Geometry: final body of the model. Coordinates: model frame, mm. A direction names the side the tool comes from. Round coordinates to 2 decimals unless told otherwise and drop trailing zeros. Write each loop counter-clockwise with the first axis right and the second up, starting at its lowest first coordinate (ties: lowest second). Pieces come first, ordered by that corner, then holes. Notation, with made-up numbers: M 42,-35 L 98,-35 A33 ccw 98,-2 Z; hole C 35.5,70 d9. An arc over 180 degrees is marked long. Answer as CSV lines item,"result". Start each with the question number.
Q1. Mould query, pull axis Y, two halves, no side actions, for faces 1 (the cylindrical face through (56.99, 17.85, 44.93)), 2 (the cylindrical face through (46.07, 38.042, 20.564)), 3 (the flat face through (15, 2, 25)). Classes: pulls with the +Y half, pulls with the -Y half, needs draft (parallel to the pull), parting line crosses it, or undercut.
Q2. Section query B-B on x = 86. Output: boundary loops of the cut face in (y, z), and give its area (3 significant figures).
Q3. Ray query, probe 1 along X at (y, z) = (3.5, 44); probe 2 along Y at (x, z) = (16, 6.5); probe 3 along Y at (x, z) = (43, 48). Return the intervals inside material, ascending.
Q4. Section query A-A on z = 4. Output: boundary loops of the cut face in (x, y).
Q5. Section query D-D on z = 42. Output: boundary loops of the cut face in (x, y).
Q6. Reachability of faces 4 (the flat face through (80, 5, 25)), 5 (the flat face through (94, 20, 6)), 6 (the flat face through (43, 28, 25)), 7 (the flat face through (80, 30, 25)) from +Z, -Z, +X, -X, +Y, -Y: full face, straight path, thin tool, end or side. Return the list, or none.
Q7. Section query C-C on y = 21.5. Output: boundary loops of the cut face in (x, z), and give its area (3 significant figures).
Q8. First-contact query: pin 1 (4.5 mm diameter, centred on x = 89.5, z = 44.5, fed in from +Y); pin 2 (23.5 mm diameter, centred on x = 45.5, y = 24.5, fed in from +Z); pin 3 (12 mm diameter, centred on x = 91.5, z = 8, fed in from +Y); pin 4 (4 mm diameter, centred on y = 26.5, z = 6, fed in from -X). Flat tips, straight axial feed; report the tip coordinate or a pass-through.
```python
from build123d import *

# Parameters (mm, degrees)
BOSS_EXTRUDE1_DEPTH = 50
BOSS_EXTRUDE2_REACH = 113.636
SKETCH2_W           = 30
SKETCH2_H           = 14.178790152
SKETCH3_R           = 10
SKETCH3_R_2         = 5
BOSS_EXTRUDE3_DEPTH = 10
SKETCH4_R           = 15
CUT_EXTRUDE1_DEPTH  = 10
SKETCH5_W           = 10
SKETCH5_H           = 5
CUT_EXTRUDE2_DEPTH  = 123.609341231


with BuildPart() as part:
    # Sketch1 → Boss-Extrude1 (new body)
    with BuildSketch(Plane.XY):
        with BuildLine():
            Line((0, 0), (0, 15))
            Line((0, 15), (50, 15))
            ThreePointArc((50, 15), (57.071067812, 17.928932188), (60, 25))
            Line((60, 25), (60, 30))
            Line((60, 30), (100, 30))
            Line((100, 30), (100, 0))
            Line((100, 0), (0, 0))
        make_face()
    extrude(amount=BOSS_EXTRUDE1_DEPTH)

    # Sketch2 → Boss-Extrude2 (add, up to next)
    with BuildSketch(Plane(origin=(7.5, -7.5, 0), x_dir=(0, 0, 1), z_dir=(-0.7071067811865488, 0.7071067811865464, 0)), mode=Mode.PRIVATE) as boss_extrude2_sk1:
        with Locations((25, 38.872545701)):
            Rectangle(SKETCH2_W, SKETCH2_H)
    boss_extrude2_tool1 = extrude(boss_extrude2_sk1.sketch, amount=-BOSS_EXTRUDE2_REACH, mode=Mode.PRIVATE) - part.part
    # Sketch2 → Boss-Extrude2 (add, up to next)
    with BuildSketch(Plane(origin=(7.5, -7.5, 0), x_dir=(0, 0, 1), z_dir=(-0.7071067811865488, 0.7071067811865464, 0)), mode=Mode.PRIVATE) as boss_extrude2_sk2:
        with BuildLine():
            Line((10, 61.783150625), (10, 45.961940777))
            Line((10, 45.961940777), (40, 45.961940777))
            Line((40, 45.961940777), (40, 61.783150625))
            ThreePointArc((40, 61.783150625), (25, 76.783150625), (10, 61.783150625))
        make_face()
    boss_extrude2_tool2 = extrude(boss_extrude2_sk2.sketch, amount=-BOSS_EXTRUDE2_REACH, mode=Mode.PRIVATE) - part.part
    add(boss_extrude2_tool1.solids().sort_by_distance((34.987041, 19.987041, 25))[0])
    add(boss_extrude2_tool2.solids().sort_by_distance((49.902416, 34.902416, 25))[0])

    # Sketch3 → Boss-Extrude3 (add)
    with BuildSketch(Plane(origin=(7.5, -7.5, 0), x_dir=(0, 0, 1), z_dir=(-0.7071067811865486, 0.7071067811865465, 0))):
        with Locations(Location((25, 61.783150625, 0), (0, 0, 270))):
            Circle(SKETCH3_R)
        with Locations(Location((25, 61.783150625, 0), (0, 0, 270))):
            Circle(SKETCH3_R_2, mode=Mode.SUBTRACT)
    extrude(amount=BOSS_EXTRUDE3_DEPTH)

    # Sketch4 → Cut-Extrude1 (cut)
    with BuildSketch(Plane(origin=(0, 30, 0), x_dir=(1, 0, 0), z_dir=(0, 1, 0))):
        with Locations((100, 0)):
            Circle(SKETCH4_R)
        with Locations((100, -50)):
            Circle(SKETCH4_R)
    extrude(amount=-CUT_EXTRUDE1_DEPTH, mode=Mode.SUBTRACT)

    # Sketch5 → Cut-Extrude2 (cut, through all)
    with BuildSketch(Plane.XY.offset(50)):
        with Locations((20, 2.5)):
            Rectangle(SKETCH5_W, SKETCH5_H)
        with Locations((80, 2.5)):
            Rectangle(SKETCH5_W, SKETCH5_H)
    extrude(amount=-CUT_EXTRUDE2_DEPTH, mode=Mode.SUBTRACT)


solid = part.part
```
Entries:
1,face 1,"pulls with the +Y half"
1,face 2,"undercut"
1,face 3,"needs draft"
2,outline,"M 0,0 L 20,0 L 20,5.39 L 30,5.39 L 30,44.61 L 20,44.61 L 20,50 L 0,50 Z"
2,area,"1,390 mm^2"
3,probe 1,"x = 0 to 15, 25 to 75, 85 to 100"
3,probe 2,"y = 5 to 15"
3,probe 3,"y = 0 to 15"
4,outline,"M 0,0 L 15,0 L 15,5 L 25,5 L 25,0 L 75,0 L 75,5 L 85,5 L 85,0 L 100,0 L 100,20 L 85.54,20 L 85.54,30 L 60,30 L 60,25 A10 cw 50,15 L 0,15 Z"
5,outline,"M 0,0 L 15,0 L 15,5 L 25,5 L 25,0 L 75,0 L 75,5 L 85,5 L 85,0 L 100,0 L 100,20 L 87.31,20 L 87.31,30 L 60,30 L 60,25 A10 cw 50,15 L 0,15 Z"
6,face 4,"+Z, -Z, -Y"
6,face 5,"-Z, +X, +Y"
6,face 6,"none"
6,face 7,"+X, +Y"
7,outline,"M 36.5,10 L 59.37,10 L 59.37,0 L 85,0 A15 cw 100,15 L 100,35 A15 cw 85,50 L 59.37,50 L 59.37,40 L 36.5,40 Z"
7,area,"2,360 mm^2"
8,pin 1,"stops at y = 20"
8,pin 2,"stops at z = 50"
8,pin 3,"stops at y = 30"
8,pin 4,"stops at x = 59.99"
